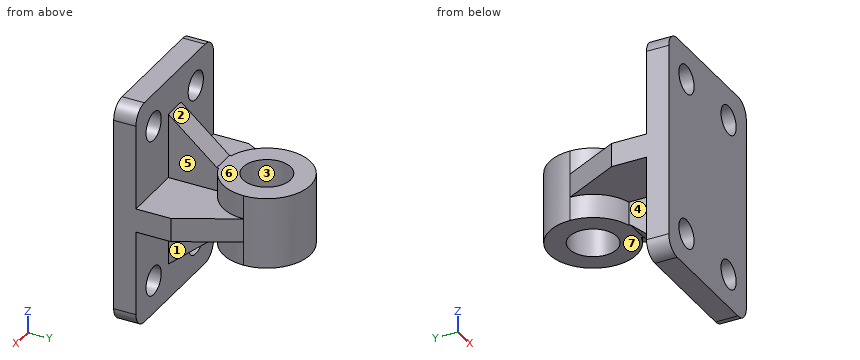
```python
from build123d import *

# Parameters (mm, degrees)
CROQUIS1_W              = 92
CROQUIS1_H              = 142
CROQUIS1_R              = 9
SALIENTE_EXTRUIR1_DEPTH = 100
CROQUIS2_R              = 15
CORTAR_EXTRUIR1_DEPTH   = 142
CORTAR_EXTRUIR2_DEPTH   = 92
CORTAR_EXTRUIR3_DEPTH   = 63.5
CORTAR_EXTRUIR4_DEPTH   = 63.5
REDONDEO1_R             = 10


with BuildPart() as part:
    # Croquis1 → Saliente-Extruir1 (new body)
    with BuildSketch(Plane(origin=(0, 0, 0), x_dir=(1, 0, 0), z_dir=(0, 1, 0))):
        with Locations((-65.401360544, 14.360544218)):
            Rectangle(CROQUIS1_W, CROQUIS1_H)
        with Locations((-90.401360544, 64.360544218)):
            Circle(CROQUIS1_R, mode=Mode.SUBTRACT)
        with Locations((-90.401360544, -35.639455782)):
            Circle(CROQUIS1_R, mode=Mode.SUBTRACT)
        with Locations((-40.401360544, 64.360544218)):
            Circle(CROQUIS1_R, mode=Mode.SUBTRACT)
        with Locations((-40.401360544, -35.639455782)):
            Circle(CROQUIS1_R, mode=Mode.SUBTRACT)
    extrude(amount=SALIENTE_EXTRUIR1_DEPTH)

    # Croquis2 → Cortar-Extruir1 (cut)
    with BuildSketch(Plane.XY.offset(56.639455782)):
        with BuildLine():
            Line((-111.401360544, 36), (-92.901360544, 72))
            ThreePointArc((-92.901360544, 72), (-65.401360544, 99.5), (-37.901360544, 72))
            Line((-37.901360544, 72), (-19.401360544, 36))
            Line((-19.401360544, 36), (-19.401360544, 100))
            Line((-19.401360544, 100), (-111.401360544, 100))
            Line((-111.401360544, 100), (-111.401360544, 36))
        make_face()
        with Locations((-65.401360544, 72)):
            Circle(CROQUIS2_R)
    extrude(amount=-CORTAR_EXTRUIR1_DEPTH, mode=Mode.SUBTRACT)

    # Croquis3 → Cortar-Extruir2 (cut)
    with BuildSketch(Plane(origin=(-19.401360544, 0, 0), x_dir=(0, 0, -1), z_dir=(1, 0, 0))):
        Polygon((62.860544218, 14), (36.860544218, 44.5), (36.860544218, 99.5), (85.360544218, 99.5), (85.360544218, 14), align=None)
        Polygon((-56.639455782, 14), (-34.139455782, 14), (-8.139455782, 44.5), (-8.139455782, 99.5), (-56.639455782, 99.5), align=None)
    extrude(amount=-CORTAR_EXTRUIR2_DEPTH, mode=Mode.SUBTRACT)

    # Croquis4 → Cortar-Extruir3 (cut)
    with BuildSketch(Plane.XY.offset(56.639455782)):
        with BuildLine():
            Line((-92.901360544, 72), (-111.401360544, 36))
            Line((-111.401360544, 36), (-111.401360544, 14))
            Line((-111.401360544, 14), (-72.901360544, 14))
            Line((-72.901360544, 14), (-72.901360544, 45.542486889))
            ThreePointArc((-72.901360544, 45.542486889), (-87.338771513, 55.416876048), (-92.901360544, 72))
        make_face()
        with BuildLine():
            Line((-19.401360544, 36), (-37.901360544, 72))
            ThreePointArc((-37.901360544, 72), (-43.463949576, 55.416876048), (-57.901360544, 45.542486889))
            Line((-57.901360544, 45.542486889), (-57.901360544, 14))
            Line((-57.901360544, 14), (-19.401360544, 14))
            Line((-19.401360544, 14), (-19.401360544, 36))
        make_face()
    extrude(amount=-CORTAR_EXTRUIR3_DEPTH, mode=Mode.SUBTRACT)

    # Croquis7 → Cortar-Extruir4 (cut)
    with BuildSketch(Plane(origin=(0, 0, -85.360544218), x_dir=(-1, 0, 0), z_dir=(0, 0, -1))):
        with BuildLine():
            Line((57.901360544, 14), (57.901360544, 45.542486889))
            ThreePointArc((57.901360544, 45.542486889), (43.463949576, 55.416876048), (37.901360544, 72))
            Line((37.901360544, 72), (19.401360544, 36))
            Line((19.401360544, 36), (19.401360544, 14))
            Line((19.401360544, 14), (57.901360544, 14))
        make_face()
        with BuildLine():
            ThreePointArc((92.901360544, 72), (87.338771513, 55.416876048), (72.901360544, 45.542486889))
            Line((72.901360544, 45.542486889), (72.901360544, 14))
            Line((72.901360544, 14), (111.401360544, 14))
            Line((111.401360544, 14), (111.401360544, 36))
            Line((111.401360544, 36), (92.901360544, 72))
        make_face()
    extrude(amount=-CORTAR_EXTRUIR4_DEPTH, mode=Mode.SUBTRACT)

    # Redondeo1
    redondeo1_edges = [part.edges().sort_by_distance(p)[0] for p in [
        (-19.401360544, 7, -85.360544218),
        (-111.401360544, 7, -85.360544218),
        (-19.401360544, 7, 56.639455782),
        (-111.401360544, 7, 56.639455782),
    ]]
    fillet(redondeo1_edges, radius=REDONDEO1_R)


solid = part.part
```
Part model, mm, in its own coordinate system. Face numbers are marked on the shaded views. A direction names the side the tool comes from. Give positions to 0.01 mm unless a question says otherwise; leave off trailing zeros. Write each loop counter-clockwise with the first axis right and the second up, starting at its lowest first coordinate (ties: lowest second). Pieces come first, ordered by that corner, then holes. Notation, with made-up numbers: M 41.5,78.5 L 58.5,78.5 A13 cw 58.5,98.5 Z; hole C 5,-12 d1. An arc over 180 degrees is marked long. Use CSV: the item, a comma, the result in double quotes.
Item 1: Slice it at C-C on x = -65.5. Write the cut outline in (y, z), plus the area to 3 significant figures.
Taken from the geometry:
outline,"M 0,-85.36 L 14,-85.36 L 14,-62.86 L 44.5,-36.86 L 57,-36.86 L 57,8.14 L 44.5,8.14 L 14,34.14 L 14,56.64 L 0,56.64 Z; M 87,-36.86 L 99.5,-36.86 L 99.5,8.14 L 87,8.14 Z"
area,"5,280 mm²"
Item 2: Pull direction X, two halves, no side cores. Call the marked faces 1, 2 and 3: +X half, -X half, draft (parallel to the pull), parting line (faces both ways), or undercut.
Taken from the geometry:
face 1,"+X half"
face 2,"draft"
face 3,"undercut"
Item 3: Slice it at B-B on x = -36. Write the cut outline in (y, z), plus the area to 3 significant figures.
Taken from the geometry:
outline,"M 0,-85.36 L 14,-85.36 L 14,-72.21 L 0,-72.21 Z; M 0,-56.51 L 14,-56.51 L 14,-21.86 L 68.3,-21.86 L 68.3,-6.86 L 14,-6.86 L 14,27.79 L 0,27.79 Z; M 0,43.49 L 14,43.49 L 14,56.64 L 0,56.64 Z"
area,"2,360 mm²"
Item 4: Slice it at D-D on z = 30. Write the cut outline in (x, y), plus the area to 3 significant figures.
Taken from the geometry:
outline,"M -111.4,0 L -97.42,0 L -97.42,14 L -111.4,14 Z; M -83.39,0 L -47.42,0 L -47.42,14 L -57.9,14 L -57.9,18.86 L -72.9,18.86 L -72.9,14 L -83.39,14 Z; M -33.39,0 L -19.4,0 L -19.4,14 L -33.39,14 Z"
area,"968 mm²"
Item 5: Drill centre lines: probe 1 along X at (y, z) = (73, -3); probe 2 along Z at (x, y) = (-89.5, 72.5); probe 3 along Z at (x, y) = (-91, 40.5). Where is each one in solid material? Low to high.
Taken from the geometry:
probe 1,"x = -92.88 to -80.37, -50.43 to -37.92"
probe 2,"z = -36.86 to 8.14"
probe 3,"z = -21.86 to -6.86"
Item 6: Slice it at A-A on z = -10.5. Write the cut outline in (x, y), plus the area to 3 significant figures.
Taken from the geometry:
outline,"M -111.4,0 L -19.4,0 L -19.4,36 L -37.9,72 A27.5 ccw -92.9,72 L -111.4,36 Z; hole C -65.4,72 d30"
area,"6,440 mm²"
Item 7: Pin check, flat tips, straight feed: P1, Ø23.5, axis at x = -90.4, z = 35.64, coming from the -Y side; P2, Ø1.5, axis at y = 30, z = 12.5, coming from the +X side; P3, Ø19, axis at x = -78, z = 31.5, coming from the +Y side; P4, Ø25, axis at y = 37.5, z = 21, coming from the -X side. Stop position of each tip, or through.
Taken from the geometry:
P1,"stops at y = 0"
P2,"stops at x = -57.9"
P3,"stops at y = 26.5"
P4,"stops at x = -72.9"
Item 8: Which spindle directions (+Z, -Z, +X, -X, +Y, -Y) get a long thin tool onto all of the face, cutting with end or side? Do the marked faces 4, 5, 6 and 7. Say none if no direction does.
Taken from the geometry:
face 4,"-Z, -X"
face 5,"+Z, +X"
face 6,"+Z, +X, -X, +Y"
face 7,"-Z, +X, -X, +Y"
